Could you check a few things on this model? Use its own coordinates, in mm. Face numbers are marked on the shaded views. A direction names the side the tool comes from. Coordinates: 2 decimals unless noted, no trailing zeros. Loops run counter-clockwise (first coordinate to the right, second up) from the corner with the lowest first, then second, coordinate; pieces in that order, holes last. Notation, with made-up numbers: (-8.5, -6) -> (36.5, -6) arc R26 cw to (36.5, 10) -> close; hole circle Ø1 at (-2, 27). An arc over 180 degrees is marked (long way). One line per question, with ' | ' between items. Start each with the question number.
(1) Suppose I cut it at D-D (z = -147.5). Please give me the cut outline in (x, y), plus the area to 3 significant figures.
(2) Which directions (+Z, -Z, +X, -X, +Y, -Y) give clear straight access to the entire face, cutting with the end or side of a thin tool? Please do the marked faces 1 and 2.
(3) Suppose I cut it at A-A (y = 42.5). Please give me the cut outline in (x, z), plus the area to 3 significant figures.
(4) Suppose I cut it at C-C (x = 88.5). Give the number of separate pieces and of enclosed holes in the cut face, plus the area to 3 significant figures.
(5) If I drill on line 1 along X through (y, z) = (62.5, -162.5); line 2 along Y through (x, z) = (44, -72); line 3 along Z through (x, y) = (42, 66), over which ranges is the centre line in solid material (lowest first)?
(6) Suppose I cut it at B-B (y = 61). Please give me the cut outline in (x, z), plus the area to 3 significant figures.
(7) I'm going to push flat-ended pins straight in: pin 1 Ø5.5 at (y, z) = (-0.5, -97) entering from +X; pin 2 Ø6 at (x, y) = (25, 61) entering from -Z; pin 3 Ø5.5 at (y, z) = (1, -75.5) entering from +X. Where does each tip first touch, or does it pass through?
(8) If we mould it in two halves opening along X, with no side actions, what happens to the marked faces 3, 4 and 5? For each: pulls with the +X half, pulls with the -X half, needs draft (parallel to the pull), parting line crosses it, or undercut.
```python
from build123d import *

# Parameters (mm, degrees)
BOSS_EXTRUDE1_DEPTH     = 3
SKETCH4_W               = 70
SKETCH4_H               = 70
BOSS_EXTRUDE3_DEPTH     = 3
SKETCH5_W               = 70
SKETCH5_H               = 70
BOSS_EXTRUDE4_DEPTH     = 3
SKETCH7_W               = 104.4
SKETCH7_H               = 70
BOSS_EXTRUDE5_DEPTH     = 5
BOSS_EXTRUDE13_DEPTH    = 2
CUT_EXTRUDE1_DEPTH      = 242.615727965
CUT_EXTRUDE1_DEPTH_BACK = 242.615727965
SKETCH26_R              = 1.35
CUT_EXTRUDE3_DEPTH      = 240.697225683
CUT_EXTRUDE3_DEPTH_BACK = 240.697225683
CUT_EXTRUDE4_DEPTH      = 223.324110253
CUT_EXTRUDE4_DEPTH_BACK = 223.324110253
SKETCH31_R              = 1.35
CUT_EXTRUDE6_DEPTH      = 5


with BuildPart() as part:
    # Sketch1 → Boss-Extrude1 (new body)
    with BuildSketch(Plane(origin=(0, 0, 0), x_dir=(1, 0, 0), z_dir=(0, 1, 0))):
        Polygon((0, 0), (104.4, 0), (129.9, 100), (129.9, 170), (-25.5, 170), (-25.5, 100), align=None)
    extrude(amount=BOSS_EXTRUDE1_DEPTH)

    # Sketch4 → Boss-Extrude3 (add)
    with BuildSketch(Plane.ZY.offset(25.5)):
        with Locations((-135, 38)):
            Rectangle(SKETCH4_W, SKETCH4_H)
    extrude(amount=-BOSS_EXTRUDE3_DEPTH)

    # Sketch5 → Boss-Extrude4 (add)
    with BuildSketch(Plane(origin=(129.9, 0, 0), x_dir=(0, 0, -1), z_dir=(1, 0, 0))):
        with Locations((135, 38)):
            Rectangle(SKETCH5_W, SKETCH5_H)
    extrude(amount=-BOSS_EXTRUDE4_DEPTH)

    # Sketch7 → Boss-Extrude5 (add)
    with BuildSketch(Plane.XY):
        with Locations((52.2, 38)):
            Rectangle(SKETCH7_W, SKETCH7_H)
    extrude(amount=-BOSS_EXTRUDE5_DEPTH)

    # Sketch22 → Boss-Extrude13 (add)
    with BuildSketch(Plane.XZ):
        Polygon((129.9, -170), (-25.5, -170), (-25.5, -100), (0, 0), (104.4, 0), (129.9, -100), align=None)
    extrude(amount=BOSS_EXTRUDE13_DEPTH)

    # Sketch26 → Cut-Extrude1 (cut, two sides: drawn at the far end of the back side and taken through both)
    with BuildSketch(Plane.ZY.offset(25.5).offset(-CUT_EXTRUDE1_DEPTH_BACK)):
        with Locations((-157.113745641, 20.7)):
            Circle(SKETCH26_R)
        with Locations((-113.113745641, 20.7)):
            Circle(SKETCH26_R)
        with Locations((-105.313745641, 27)):
            Circle(SKETCH26_R)
        with Locations((-105.313745641, 49)):
            Circle(SKETCH26_R)
        with Locations((-113.113745641, 55.3)):
            Circle(SKETCH26_R)
        with Locations((-135.113745641, 55.3)):
            Circle(SKETCH26_R)
        with Locations((-157.113745641, 55.3)):
            Circle(SKETCH26_R)
        with Locations((-135.113745641, 20.7)):
            Circle(SKETCH26_R)
    extrude(amount=CUT_EXTRUDE1_DEPTH + CUT_EXTRUDE1_DEPTH_BACK, mode=Mode.SUBTRACT)

    # Sketch28 → Cut-Extrude3 (cut, two sides: drawn at the far end of the back side and taken through both)
    with BuildSketch(Plane(origin=(-22.5, 0, 0), x_dir=(0, 0, -1), z_dir=(1, 0, 0)).offset(-CUT_EXTRUDE3_DEPTH_BACK)):
        with BuildLine():
            Line((167.613745641, 49.5), (167.613745641, 26.5))
            ThreePointArc((167.613745641, 26.5), (166.735065984, 24.378679656), (164.613745641, 23.5))
            Line((164.613745641, 23.5), (111.113745641, 23.5))
            ThreePointArc((111.113745641, 23.5), (108.992425297, 24.378679656), (108.113745641, 26.5))
            Line((108.113745641, 26.5), (108.113745641, 49.5))
            ThreePointArc((108.113745641, 49.5), (108.992425297, 51.621320344), (111.113745641, 52.5))
            Line((111.113745641, 52.5), (164.613745641, 52.5))
            ThreePointArc((164.613745641, 52.5), (166.735065984, 51.621320344), (167.613745641, 49.5))
        make_face()
    extrude(amount=CUT_EXTRUDE3_DEPTH + CUT_EXTRUDE3_DEPTH_BACK, mode=Mode.SUBTRACT)

    # Sketch31 → Cut-Extrude4 (cut, two sides: drawn at the far end of the back side and taken through both)
    with BuildSketch(Plane(origin=(0, 0, -5), x_dir=(-1, 0, 0), z_dir=(0, 0, -1)).offset(-CUT_EXTRUDE4_DEPTH_BACK)):
        with BuildLine():
            Line((0, 52.5), (-36.563880863, 52.5))
            ThreePointArc((-36.563880863, 52.5), (-38.685201207, 51.621320344), (-39.563880863, 49.5))
            Line((-39.563880863, 49.5), (-39.563880863, 26.5))
            ThreePointArc((-39.563880863, 26.5), (-38.685201207, 24.378679656), (-36.563880863, 23.5))
            Line((-36.563880863, 23.5), (0, 23.5))
            Line((0, 23.5), (0, 25.098503624))
            ThreePointArc((0, 25.098503624), (-8.563880863, 38), (0, 50.901496376))
            Line((0, 50.901496376), (0, 52.5))
        make_face()
        with BuildLine():
            Line((0, 25.098503624), (0, 50.901496376))
            ThreePointArc((0, 50.901496376), (-8.563880863, 38), (0, 25.098503624))
        make_face()
        with BuildLine():
            ThreePointArc((-67.836119137, 23.5), (-65.714798793, 24.378679656), (-64.836119137, 26.5))
            Line((-64.836119137, 26.5), (-64.836119137, 49.5))
            ThreePointArc((-64.836119137, 49.5), (-65.714798793, 51.621320344), (-67.836119137, 52.5))
            Line((-67.836119137, 52.5), (-104.4, 52.5))
            Line((-104.4, 52.5), (-104.4, 50.901496376))
            ThreePointArc((-104.4, 50.901496376), (-95.836119137, 38), (-104.4, 25.098503624))
            Line((-104.4, 25.098503624), (-104.4, 23.5))
            Line((-104.4, 23.5), (-67.836119137, 23.5))
        make_face()
        with BuildLine():
            Line((-104.4, 50.901496376), (-104.4, 25.098503624))
            ThreePointArc((-104.4, 25.098503624), (-95.836119137, 38), (-104.4, 50.901496376))
        make_face()
        with Locations(Location((-91.836119137, 20.7, 0), (0, 0, 180))):
            Circle(SKETCH31_R)
        with Locations(Location((-69.836119137, 20.7, 0), (0, 0, 180))):
            Circle(SKETCH31_R)
        with Locations(Location((-62.036119137, 27, 0), (0, 0, 180))):
            Circle(SKETCH31_R)
        with Locations(Location((-62.036119137, 49, 0), (0, 0, 180))):
            Circle(SKETCH31_R)
        with Locations(Location((-69.836119137, 55.3, 0), (0, 0, 180))):
            Circle(SKETCH31_R)
        with Locations(Location((-91.836119137, 55.3, 0), (0, 0, 180))):
            Circle(SKETCH31_R)
        with Locations((-34.563880863, 55.3)):
            Circle(SKETCH31_R)
        with Locations((-42.363880863, 49)):
            Circle(SKETCH31_R)
        with Locations((-42.363880863, 27)):
            Circle(SKETCH31_R)
        with Locations((-34.563880863, 20.7)):
            Circle(SKETCH31_R)
        with Locations((-12.563880863, 20.7)):
            Circle(SKETCH31_R)
        with Locations((-12.563880863, 55.3)):
            Circle(SKETCH31_R)
    extrude(amount=CUT_EXTRUDE4_DEPTH + CUT_EXTRUDE4_DEPTH_BACK, mode=Mode.SUBTRACT)

    # Sketch32 → Cut-Extrude6 (cut)
    with BuildSketch(Plane(origin=(0, -2, 0), x_dir=(-1, 0, 0), z_dir=(0, -1, 0))):
        Polygon((-62.2, 142.065285868), (-62.2, 152.065285868), (-107.2, 160), (-107.2, 150), align=None)
        Polygon((-52.2, 140.302016061), (-52.2, 150.302016061), (-62.2, 152.065285868), (-62.2, 142.065285868), align=None)
        Polygon((-42.2, 152.065285868), (-52.2, 150.302016061), (-52.2, 140.302016061), (-42.2, 142.065285868), align=None)
        Polygon((2.8, 160), (-42.2, 152.065285868), (-42.2, 142.065285868), (2.8, 150), align=None)
        Polygon((-62.2, 122.065285868), (-62.2, 132.065285868), (-107.2, 140), (-107.2, 130), align=None)
        Polygon((-52.2, 120.302016061), (-52.2, 130.302016061), (-62.2, 132.065285868), (-62.2, 122.065285868), align=None)
        Polygon((-42.2, 132.065285868), (-52.2, 130.302016061), (-52.2, 120.302016061), (-42.2, 122.065285868), align=None)
        Polygon((2.8, 140), (-42.2, 132.065285868), (-42.2, 122.065285868), (2.8, 130), align=None)
        Polygon((-62.2, 102.065285868), (-62.2, 112.065285868), (-107.2, 120), (-107.2, 110), align=None)
        Polygon((-52.2, 100.302016061), (-52.2, 110.302016061), (-62.2, 112.065285868), (-62.2, 102.065285868), align=None)
        Polygon((-42.2, 112.065285868), (-52.2, 110.302016061), (-52.2, 100.302016061), (-42.2, 102.065285868), align=None)
        Polygon((2.8, 120), (-42.2, 112.065285868), (-42.2, 102.065285868), (2.8, 110), align=None)
        Polygon((-62.2, 82.065285868), (-62.2, 92.065285868), (-107.2, 100), (-107.2, 90), align=None)
        Polygon((-52.2, 80.302016061), (-52.2, 90.302016061), (-62.2, 92.065285868), (-62.2, 82.065285868), align=None)
        Polygon((-42.2, 92.065285868), (-52.2, 90.302016061), (-52.2, 80.302016061), (-42.2, 82.065285868), align=None)
        Polygon((2.8, 100), (-42.2, 92.065285868), (-42.2, 82.065285868), (2.8, 90), align=None)
        Polygon((-62.2, 62.065285868), (-62.2, 72.065285868), (-107.2, 80), (-107.2, 70), align=None)
        Polygon((-52.2, 60.302016061), (-52.2, 70.302016061), (-62.2, 72.065285868), (-62.2, 62.065285868), align=None)
        Polygon((-42.2, 72.065285868), (-52.2, 70.302016061), (-52.2, 60.302016061), (-42.2, 62.065285868), align=None)
        Polygon((2.8, 80), (-42.2, 72.065285868), (-42.2, 62.065285868), (2.8, 70), align=None)
        Polygon((-62.2, 42.065285868), (-62.2, 52.065285868), (-107.2, 60), (-107.2, 50), align=None)
        Polygon((-52.2, 40.302016061), (-52.2, 50.302016061), (-62.2, 52.065285868), (-62.2, 42.065285868), align=None)
        Polygon((-42.2, 52.065285868), (-52.2, 50.302016061), (-52.2, 40.302016061), (-42.2, 42.065285868), align=None)
        Polygon((2.8, 60), (-42.2, 52.065285868), (-42.2, 42.065285868), (2.8, 50), align=None)
        Polygon((-52.2, 30.302016061), (-52.2, 40.302016061), (-62.2, 42.065285868), (-62.2, 32.065285868), align=None)
        Polygon((-42.2, 42.065285868), (-52.2, 40.302016061), (-52.2, 30.302016061), (-42.2, 32.065285868), align=None)
        Polygon((-42.2, 32.065285868), (-52.2, 30.302016061), (-52.2, 20.302016061), (-42.2, 22.065285868), align=None)
        Polygon((-52.2, 20.302016061), (-52.2, 30.302016061), (-62.2, 32.065285868), (-62.2, 22.065285868), align=None)
    extrude(amount=-CUT_EXTRUDE6_DEPTH, mode=Mode.SUBTRACT)


solid = part.part
```
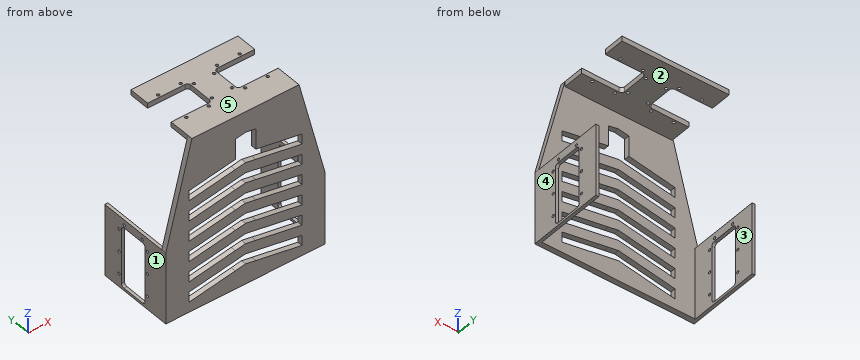
Checks:
1) outline: (-25.5, -2) -> (11.38, -2) -> (11.38, 3) -> (-22.5, 3) -> (-22.5, 23.5) -> (-25.5, 23.5) -> close; (-25.5, 52.5) -> (-22.5, 52.5) -> (-22.5, 73) -> (-25.5, 73) -> close; (93.02, -2) -> (129.9, -2) -> (129.9, 23.5) -> (126.9, 23.5) -> (126.9, 3) -> (93.02, 3) -> close; (126.9, 52.5) -> (129.9, 52.5) -> (129.9, 73) -> (126.9, 73) -> close | area: 615 mm^2
2) face 1: +Z, -Z, -X, +Y, -Y | face 2: -Z, +X, -X, +Y
3) outline: (-25.5, -170) -> (-22.5, -170) -> (-22.5, -167.61) -> (-25.5, -167.61) -> close; (-25.5, -108.11) -> (-22.5, -108.11) -> (-22.5, -100) -> (-25.5, -100) -> close; (39.56, -5) -> (64.84, -5) -> (64.84, 0) -> (39.56, 0) -> close; (126.9, -170) -> (129.9, -170) -> (129.9, -167.61) -> (126.9, -167.61) -> close; (126.9, -108.11) -> (129.9, -108.11) -> (129.9, -100) -> (126.9, -100) -> close | area: 189 mm^2
4) separate pieces: 8 | enclosed holes: 0 | area: 755 mm^2
5) line 1: x = -25.5 to -22.5, 126.9 to 129.9 | line 2: y = -2 to 3 | line 3: z = -5 to 0
6) outline: (-25.5, -170) -> (-22.5, -170) -> (-22.5, -100) -> (-25.5, -100) -> close; (0, -5) -> (104.4, -5) -> (104.4, 0) -> (0, 0) -> close; (126.9, -170) -> (129.9, -170) -> (129.9, -100) -> (126.9, -100) -> close | area: 942 mm^2
7) pin 1: stops at x = 129.84 | pin 2: stops at z = -5 | pin 3: stops at x = 124.35
8) face 3: undercut | face 4: pulls with the +X half | face 5: needs draft
